Geometry check sheet. Reference: drawing and pictorial views, mm from the part's lowest x, y, z. A direction names the side the tool comes from. Round coordinates to 2 decimals unless told otherwise and drop trailing zeros. Order: outer loops, then holes, each group sorted by start corner. A loop starts at its lowest first (then second) coordinate and runs counter-clockwise, first axis right, second up.
(1) Draft check along Z on the marked faces 3, 4 and 5. Enter one of: pulls with the +Z half, pulls with the -Z half, needs draft (parallel to the pull), parting line crosses it, or undercut.
(2) Cross-section at C-C on x = 58.5. Enter the section's corners in (y, z), and give its area (3 significant figures).
(3) Thickness scan on L1, parallel to Z at x = 50.5, y = 4.5; L2, parallel to Z at x = 47.5, y = 1.75; L3, parallel to X at y = 12.25, z = 74. Record the ranges inside material, lowest first.
(4) Cross-section at D-D on z = 23.5. Enter the section's corners in (x, y), and give its area (3 significant figures).
(5) Gauge pin test, flat end, axial feed: P1, Ø4, axis at y = 4, z = 56.5, coming from the +X side. Record the tip position at first contact, or that the pin passes through.
(6) Cross-section at A-A on z = 56. Enter the section's corners in (x, y).
(7) Cross-section at B-B on y = 7.5. Enter the section's corners in (x, z) (1 decimal).
(8) Set-up check for the marked faces 1 and 2: record each of +Z, -Z, +X, -X, +Y, -Y from which the full face is reachable in a straight line by a thin tool's end or side.
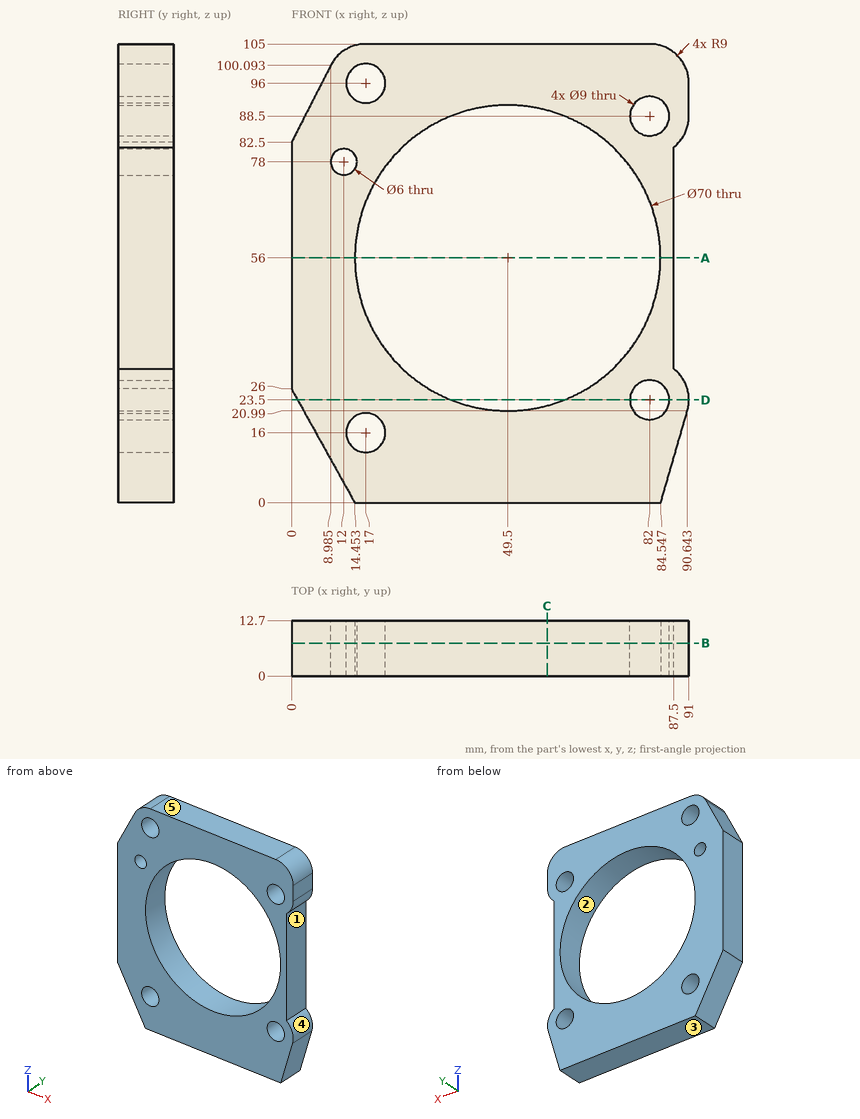
Found:
1. face 3: pulls with the -Z half
1. face 4: undercut
1. face 5: pulls with the +Z half
2. outline: (0, 0) - (12.7, 0) - (12.7, 22.18) - (0, 22.18) - close; (0, 89.82) - (12.7, 89.82) - (12.7, 105) - (0, 105) - close
2. area: 474 mm2
3. L1: z = 0 to 21.01, 90.99 to 105
3. L2: z = 0 to 21.06, 90.94 to 105
3. L3: x = 0 to 19.48, 79.52 to 87.5
4. outline: (1.39, 0) - (36.51, 0) - (36.51, 12.7) - (1.39, 12.7) - close; (62.49, 0) - (77.5, 0) - (77.5, 12.7) - (62.49, 12.7) - close; (86.5, 0) - (91, 0) - (91, 12.7) - (86.5, 12.7) - close
4. area: 694 mm2
5. P1: stops at x = 87.5
6. outline: (0, 0) - (14.5, 0) - (14.5, 12.7) - (0, 12.7) - close; (84.5, 0) - (87.5, 0) - (87.5, 12.7) - (84.5, 12.7) - close
7. outline: (0, 26) - (14.5, 0) - (84.5, 0) - (90.6, 21) arc R9 ccw to (87.5, 30.6) - (87.5, 81.4) arc R9 ccw to (91, 88.5) - (91, 96) arc R9 ccw to (82, 105) - (17, 105) arc R9 ccw to (9, 100.1) - (0, 82.5) - close; hole circle Ø6 at (12, 78); hole circle Ø9 at (17, 16); hole circle Ø9 at (17, 96); hole circle Ø70 at (49.5, 56); hole circle Ø9 at (82, 23.5); hole circle Ø9 at (82, 88.5)
8. face 1: +X, +Y, -Y
8. face 2: +Y, -Y
